Read the model definition and answer for the solid it produces. Units are mm, in the model's axes. Coordinates: 2 decimals unless noted, no trailing zeros. Write each loop counter-clockwise with the first axis right and the second up, starting at its lowest first coordinate (ties: lowest second). Pieces come first, ordered by that corner, then holes.
(1) The part is cut by section A-A, the plane x = 35. Determine the outline of the cut face in (y, z).
(2) The part is cut by section B-B, the plane z = 5.25. Determine the outline of the cut face in (x, y), and give its area (3 significant figures).
(3) Given pin 1 (5 mm diameter, centred on x = 52.5, y = -52.5, fed in from -Z), flat-ended and moving along its own axis, determine where the tip first touches the part or whether it passes through.
(4) Determine the mould class of faces 1 (the cylindrical face through (17.24, -15.517, 5.07)), 2 (the flat face through (35, -57, 10)), 3 (the flat face through (35, 0, 5)) for opening direction Y: pulls with the +Y half, pulls with the -Y half, needs draft (parallel to the pull), parting line crosses it, or undercut.
(5) Straight lines are drawn through the part: line 1 along Y through (x, z) = (35, 6.25); line 2 along Y through (x, z) = (28, 7.5); line 3 along X through (y, z) = (-46, 1.5). For each, find the intervals that lie inside material, in ascending order.
(6) The part is cut by section C-C, the plane y = -35. Determine the outline of the cut face in (x, z), and give its area (3 significant figures).
```python
from build123d import *

# Parameters (mm, degrees)
SKETCH1_W           = 70
SKETCH1_H           = 80
SKETCH1_R           = 17.5
BOSS_EXTRUDE1_DEPTH = 10
FILLET1_R           = 20
SKETCH2_R           = 2
CUT_EXTRUDE1_DEPTH  = 10


with BuildPart() as part:
    # Sketch1 → Boss-Extrude1 (new body)
    with BuildSketch(Plane.XY):
        with Locations((35, -40)):
            Rectangle(SKETCH1_W, SKETCH1_H)
        with Locations((35, -35)):
            Circle(SKETCH1_R, mode=Mode.SUBTRACT)
    extrude(amount=BOSS_EXTRUDE1_DEPTH)

    # Fillet1
    fillet1_edges = [part.edges().sort_by_distance(p)[0] for p in [
        (0, 0, 5),
        (70, 0, 5),
    ]]
    fillet(fillet1_edges, radius=FILLET1_R)

    # Sketch2 → Cut-Extrude1 (cut)
    with BuildSketch(Plane.XY.offset(10)):
        with Locations((17.5, -17.5)):
            Circle(SKETCH2_R)
        with Locations((52.5, -17.5)):
            Circle(SKETCH2_R)
        with Locations((52.5, -52.5)):
            Circle(SKETCH2_R)
        with Locations((17.5, -52.5)):
            Circle(SKETCH2_R)
    extrude(amount=-CUT_EXTRUDE1_DEPTH, mode=Mode.SUBTRACT)


solid = part.part
```
Computed:
1. outline: (-80, 0) - (-52.5, 0) - (-52.5, 10) - (-80, 10) - close; (-17.5, 0) - (0, 0) - (0, 10) - (-17.5, 10) - close
2. outline: (0, -80) - (70, -80) - (70, -20) arc R20 ccw to (50, 0) - (20, 0) arc R20 ccw to (0, -20) - close; hole circle Ø4 at (17.5, -52.5); hole circle Ø4 at (17.5, -17.5); hole circle Ø35 at (35, -35); hole circle Ø4 at (52.5, -52.5); hole circle Ø4 at (52.5, -17.5)
2. area: 4,420 mm2
3. pin 1: stops at z = 0
4. face 1: undercut
4. face 2: needs draft
4. face 3: pulls with the +Y half
5. line 1: y = -80 to -52.5, -17.5 to 0
5. line 2: y = -80 to -51.04, -18.96 to 0
5. line 3: x = 0 to 21.39, 48.61 to 70
6. outline: (0, 0) - (17.5, 0) - (17.5, 10) - (0, 10) - close; (52.5, 0) - (70, 0) - (70, 10) - (52.5, 10) - close
6. area: 350 mm2
